Design review of the part built by this model. Coordinates are the model's own, in mm. Coordinates: 2 decimals unless noted, no trailing zeros. Write each loop counter-clockwise with the first axis right and the second up, starting at its lowest first coordinate (ties: lowest second). Pieces come first, ordered by that corner, then holes.
Q1. For pin 1 Ø3 at (x, z) = (325.5, 4) entering from +Y, flat-tipped, find the tip position at first contact; note if it passes through.
Q2. For L1, parallel to Y at x = 172.75, z = 4; L2, parallel to X at y = 82.5, z = 4.25; L3, parallel to Y at x = 322, z = 3.5, list the stretches that pass through material, from the lowest coordinate up.
Q3. Take a section at B-B, the plane z = 5.5. State how many separate pieces and enclosed holes the cut face has, plus the area to 3 significant figures.
Q4. Take a section at A-A, the plane x = 60. Write out the cut boundary in (y, z).
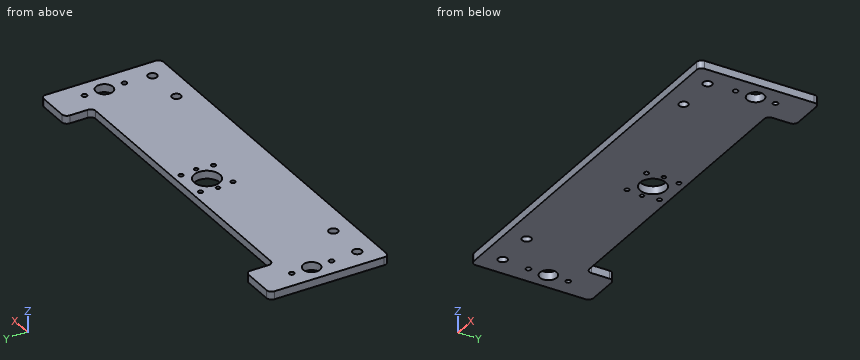
from build123d import *

# Parameters (mm, degrees)
F0_R     = 4.5
F0_R_2   = 2.5
F0_R_3   = 2.25
F0_R_4   = 8.5
F0_R_5   = 2
F0_R_6   = 13
F1_DEPTH = 8
F2_DEPTH = 25
F3_R     = 5


with BuildPart() as f1:
    # F0 (on Top) → F1 (new body)
    with BuildSketch(Plane.XY):
        Polygon((0, 120), (0, 0), (382, 0), (382, 120), (342, 120), (342, 92), (40, 92), (40, 120), align=None)
        with Locations((20, 20)):
            Circle(F0_R, mode=Mode.SUBTRACT)
        with Locations((60, 20)):
            Circle(F0_R, mode=Mode.SUBTRACT)
        with Locations((18, 47)):
            Circle(F0_R_2, mode=Mode.SUBTRACT)
        with Locations((174.736544, 51.736544)):
            Circle(F0_R_3, mode=Mode.SUBTRACT)
        with Locations((322, 20)):
            Circle(F0_R, mode=Mode.SUBTRACT)
        with Locations((362, 20)):
            Circle(F0_R, mode=Mode.SUBTRACT)
        with Locations((207.263456, 51.736544)):
            Circle(F0_R_3, mode=Mode.SUBTRACT)
        with Locations((364, 47)):
            Circle(F0_R_2, mode=Mode.SUBTRACT)
        with Locations((18, 67)):
            Circle(F0_R_4, mode=Mode.SUBTRACT)
        with Locations((18, 87)):
            Circle(F0_R_2, mode=Mode.SUBTRACT)
        with Locations((172.75, 68)):
            Circle(F0_R_5, mode=Mode.SUBTRACT)
        with Locations((174.736544, 84.263456)):
            Circle(F0_R_3, mode=Mode.SUBTRACT)
        with Locations((191, 68)):
            Circle(F0_R_6, mode=Mode.SUBTRACT)
        with Locations((209.25, 68)):
            Circle(F0_R_5, mode=Mode.SUBTRACT)
        with Locations((207.263456, 84.263456)):
            Circle(F0_R_3, mode=Mode.SUBTRACT)
        with Locations((364, 67)):
            Circle(F0_R_4, mode=Mode.SUBTRACT)
        with Locations((364, 87)):
            Circle(F0_R_2, mode=Mode.SUBTRACT)
    extrude(amount=F1_DEPTH)

    # F0 (on Top) → F2 (cut)
    with BuildSketch(Plane.XY):
        Polygon((0, 120), (0, 0), (382, 0), (382, 120), (342, 120), (342, 92), (40, 92), (40, 120), align=None)
        with Locations((20, 20)):
            Circle(F0_R, mode=Mode.SUBTRACT)
        with Locations((60, 20)):
            Circle(F0_R, mode=Mode.SUBTRACT)
        with Locations((18, 47)):
            Circle(F0_R_2, mode=Mode.SUBTRACT)
        with Locations((174.736544, 51.736544)):
            Circle(F0_R_3, mode=Mode.SUBTRACT)
        with Locations((322, 20)):
            Circle(F0_R, mode=Mode.SUBTRACT)
        with Locations((362, 20)):
            Circle(F0_R, mode=Mode.SUBTRACT)
        with Locations((207.263456, 51.736544)):
            Circle(F0_R_3, mode=Mode.SUBTRACT)
        with Locations((364, 47)):
            Circle(F0_R_2, mode=Mode.SUBTRACT)
        with Locations((18, 67)):
            Circle(F0_R_4, mode=Mode.SUBTRACT)
        with Locations((18, 87)):
            Circle(F0_R_2, mode=Mode.SUBTRACT)
        with Locations((172.75, 68)):
            Circle(F0_R_5, mode=Mode.SUBTRACT)
        with Locations((174.736544, 84.263456)):
            Circle(F0_R_3, mode=Mode.SUBTRACT)
        with Locations((191, 68)):
            Circle(F0_R_6, mode=Mode.SUBTRACT)
        with Locations((209.25, 68)):
            Circle(F0_R_5, mode=Mode.SUBTRACT)
        with Locations((207.263456, 84.263456)):
            Circle(F0_R_3, mode=Mode.SUBTRACT)
        with Locations((364, 67)):
            Circle(F0_R_4, mode=Mode.SUBTRACT)
        with Locations((364, 87)):
            Circle(F0_R_2, mode=Mode.SUBTRACT)
    extrude(amount=-F2_DEPTH, mode=Mode.SUBTRACT)

    # F3
    f3_edges = [f1.edges().sort_by_distance(p)[0] for p in [
        (382, 0, 4),
        (382, 120, 4),
        (342, 120, 4),
        (342, 92, 4),
        (40, 92, 4),
        (40, 120, 4),
        (0, 120, 4),
        (0, 0, 4),
    ]]
    fillet(f3_edges, radius=F3_R)


solid = f1.part
Responses:
1. pin 1: stops at y = 92
2. L1: y = 0 to 50.68, 52.79 to 66, 70 to 83.21, 85.32 to 92
2. L2: x = 0 to 173.34, 176.13 to 205.87, 208.66 to 382
2. L3: y = 0 to 15.5, 24.5 to 92
3. separate pieces: 1
3. enclosed holes: 17
3. area: 36,000 mm2
4. outline: (0, 0) - (15.5, 0) - (15.5, 8) - (0, 8) - close; (24.5, 0) - (92, 0) - (92, 8) - (24.5, 8) - close
